Drawing for the job (mm, zero at the part's lowest x, y, z). Round coordinates to 2 decimals unless told otherwise and drop trailing zeros. Loops run counter-clockwise (first coordinate to the right, second up) from the corner with the lowest first, then second, coordinate; pieces in that order, holes last. Notation, with made-up numbers: (-40, 60.5) - (-35, 60.5) arc R10 cw to (-35, 67.5) - close; hole circle Ø7 at (19, -16.5). An arc over 180 degrees is marked (long way). Put each result on its own line as item: value.
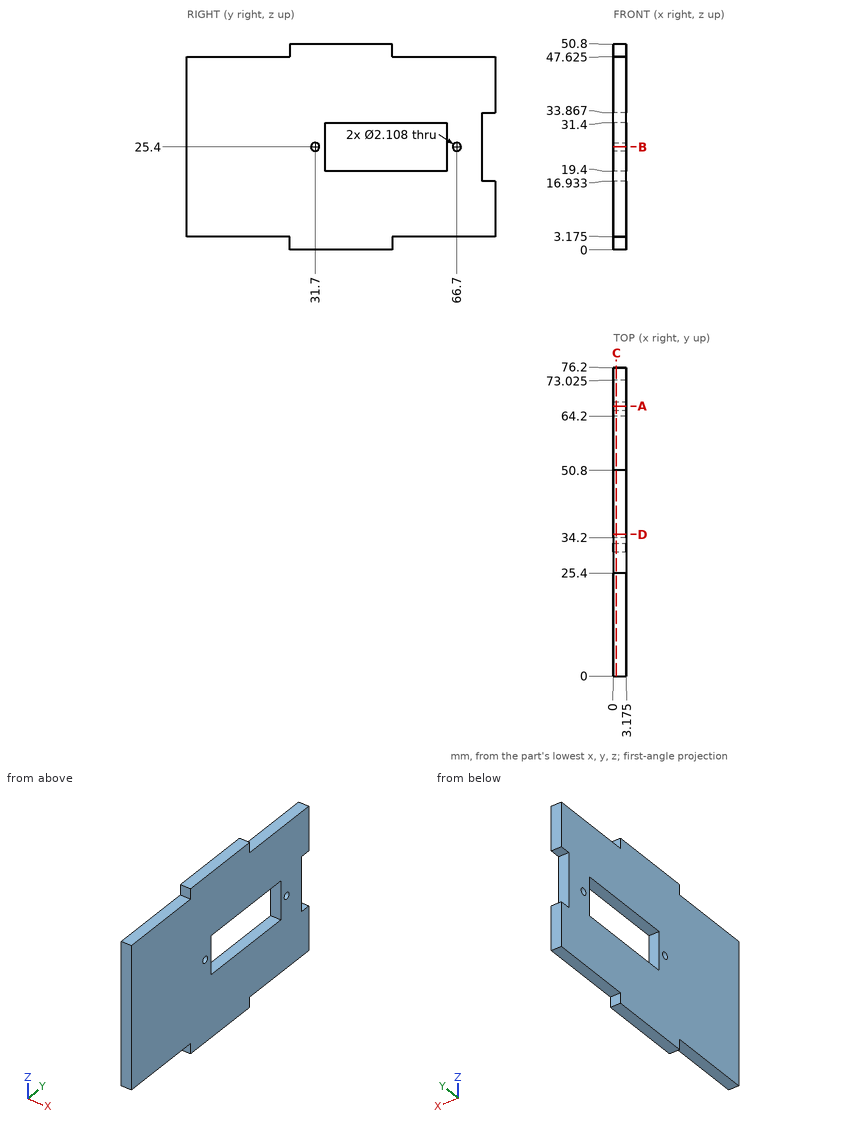
1. Probe line 1 along Y through (x, z) = (2.5, 25.4) (1 decimal); line 2 along Z through (x, y) = (0.65, 57.5) (1 decimal); line 3 along Z through (x, y) = (1.9, 66.7) (1 decimal). List the from-to ranges inside material, lowest first. Write a range as [from, to].
A:
line 1: y = [0, 30.6], [32.8, 34.2], [64.2, 65.6], [67.8, 73]
line 2: z = [3.2, 19.4], [31.4, 47.6]
line 3: z = [3.2, 24.3], [26.5, 47.6]
2. Band-saw the part on A-A (y = 66.7). List the corners of the cut face in (x, z) (1 decimal).
A:
outline: (0, 3.2) - (3.2, 3.2) - (3.2, 24.3) - (0, 24.3) - close; (0, 26.5) - (3.2, 26.5) - (3.2, 47.6) - (0, 47.6) - close
3. Pin check, flat tips, straight feed: P1, Ø1.6, axis at x = 2, y = 15, coming from the -Z side (3 decimals); P2, Ø1, axis at x = 1.5, z = 1.5, coming from the +Y side; P3, Ø1.6, axis at x = 1.5, y = 62.5, coming from the +Z side (3 decimals). Stop position of each tip, or through.
A:
P1: stops at z = 3.175
P2: stops at y = 50.8
P3: stops at z = 47.625
4. Band-saw the part on C-C (x = 0.75). List the corners of the cut face in (y, z) (1 decimal).
A:
outline: (0, 3.2) - (25.4, 3.2) - (25.4, 0) - (50.8, 0) - (50.8, 3.2) - (76.2, 3.2) - (76.2, 16.9) - (73, 16.9) - (73, 33.9) - (76.2, 33.9) - (76.2, 47.6) - (50.8, 47.6) - (50.8, 50.8) - (25.4, 50.8) - (25.4, 47.6) - (0, 47.6) - close; hole circle Ø2.1 at (31.7, 25.4); hole (34.2, 19.4) - (64.2, 19.4) - (64.2, 31.4) - (34.2, 31.4) - close; hole circle Ø2.1 at (66.7, 25.4)
5. Band-saw the part on D-D (y = 35). List the corners of the cut face in (x, z) (1 decimal).
A:
outline: (0, 0) - (3.2, 0) - (3.2, 19.4) - (0, 19.4) - close; (0, 31.4) - (3.2, 31.4) - (3.2, 50.8) - (0, 50.8) - close
6. Band-saw the part on B-B (z = 25.4). List the corners of the cut face in (x, y) (1 decimal).
A:
outline: (0, 0) - (3.2, 0) - (3.2, 30.6) - (0, 30.6) - close; (0, 32.8) - (3.2, 32.8) - (3.2, 34.2) - (0, 34.2) - close; (0, 64.2) - (3.2, 64.2) - (3.2, 65.6) - (0, 65.6) - close; (0, 67.8) - (3.2, 67.8) - (3.2, 73) - (0, 73) - close
